```python
from build123d import *

# Parameters (mm, degrees)
F0_W     = 152.4
F0_H     = 101.6
F0_R     = 25.4
F1_DEPTH = 50.8
F2_R     = 5.08
F3_R     = 5.08
F4_R     = 5.08
F5_R     = 5.08
F6_SIZE  = 5.08


with BuildPart() as f1:
    # F0 (on Top) → F1 (new body)
    with BuildSketch(Plane.XY):
        Rectangle(F0_W, F0_H)
        Circle(F0_R, mode=Mode.SUBTRACT)
    extrude(amount=F1_DEPTH)

    # F2
    f2_edges = [f1.edges().sort_by_distance(p)[0] for p in [
        (0, -50.8, 50.8),
    ]]
    fillet(f2_edges, radius=F2_R)

    # F3
    f3_edges = [f1.edges().sort_by_distance(p)[0] for p in [
        (76.2, 2.54, 50.8),
    ]]
    fillet(f3_edges, radius=F3_R)

    # F4
    f4_edges = [f1.edges().sort_by_distance(p)[0] for p in [
        (-76.2, 2.54, 50.8),
    ]]
    fillet(f4_edges, radius=F4_R)

    # F5
    f5_edges = [f1.edges().sort_by_distance(p)[0] for p in [
        (-71.12, 2.54, 50.8),
        (0, 50.8, 50.8),
    ]]
    fillet(f5_edges, radius=F5_R)

    # F6
    f6_edges = [f1.edges().sort_by_distance(p)[0] for p in [
        (-25.4, 0, 50.8),
    ]]
    chamfer(f6_edges, length=F6_SIZE)


solid = f1.part
```
Geometry: final body of the model. Coordinates: model frame, mm. Coordinates: 2 decimals unless noted, no trailing zeros. Order: outer loops, then holes, each group sorted by start corner. A loop starts at its lowest first (then second) coordinate and runs counter-clockwise, first axis right, second up. Notation, with made-up numbers: M 47,47.5 L 91,47.5 A22 ccw 91,73.5 Z; hole C 34,39.5 d2. An arc over 180 degrees is marked long. Answer in a Markdown table with one row per item. Add a question column.
Q1. Mould query, pull axis X, two halves, no side actions, for faces 1 (the cylindrical face through (-5.506, -24.796, 22.54)), 2 (the cylindrical face through (0.996, 49.272, 49.351)), 3 (the flat face through (-76.2, -1, 23)). Classes: released by +X, released by -X, zero draft, split by the parting line, or undercut.
Q2. Section query B-B on x = 0. Return the cut outline in (y, z).
Q3. Section query A-A on y = 0. Return the cut outline in (x, z), and give its area (3 significant figures).
Q4. Section query C-C on z = 9. Return the cut outline in (x, y), and give its area (3 significant figures).
Q5. Contact query for a flat-ended pin moving along its axis: P1, Ø1.5, axis at x = -49.5, y = 30, coming from the -Z side. Output: stop coordinate, or through.
Q6. Line query: L1, parallel to Y at x = 0, z = 13.5; L2, parallel to X at y = 18, z = 48; L3, parallel to X at y = -3.5, z = 6. Output: solid intervals per line, ascending.
Completed:
| question | item | result |
|---|---|---|
| 1 | face 1 | undercut |
| 1 | face 2 | zero draft |
| 1 | face 3 | released by -X |
| 2 | outline | M -50.8,0 L -25.4,0 L -25.4,45.72 L -30.48,50.8 L -45.72,50.8 A5.08 ccw -50.8,45.72 Z; M 25.4,0 L 50.8,0 L 50.8,45.72 A5.08 ccw 45.72,50.8 L 30.48,50.8 L 25.4,45.72 Z |
| 3 | outline | M -76.2,0 L -25.4,0 L -25.4,45.72 L -30.48,50.8 L -71.12,50.8 A5.08 ccw -76.2,45.72 Z; M 25.4,0 L 76.2,0 L 76.2,45.72 A5.08 ccw 71.12,50.8 L 30.48,50.8 L 25.4,45.72 Z |
| 3 | area | 5,120 mm2 |
| 4 | outline | M -76.2,-45.72 A5.08 ccw -71.12,-50.8 L 71.12,-50.8 A5.08 ccw 76.2,-45.72 L 76.2,45.72 A5.08 ccw 71.12,50.8 L -71.12,50.8 A5.08 ccw -76.2,45.72 Z; hole C 0,0 d50.8 |
| 4 | area | 13,400 mm2 |
| 5 | P1 | stops at z = 0 |
| 6 | L1 | y = -50.8 to -25.4, 25.4 to 50.8 |
| 6 | L2 | x = -75.66 to -21.03, 21.03 to 75.66 |
| 6 | L3 | x = -76.2 to -25.16, 25.16 to 76.2 |
